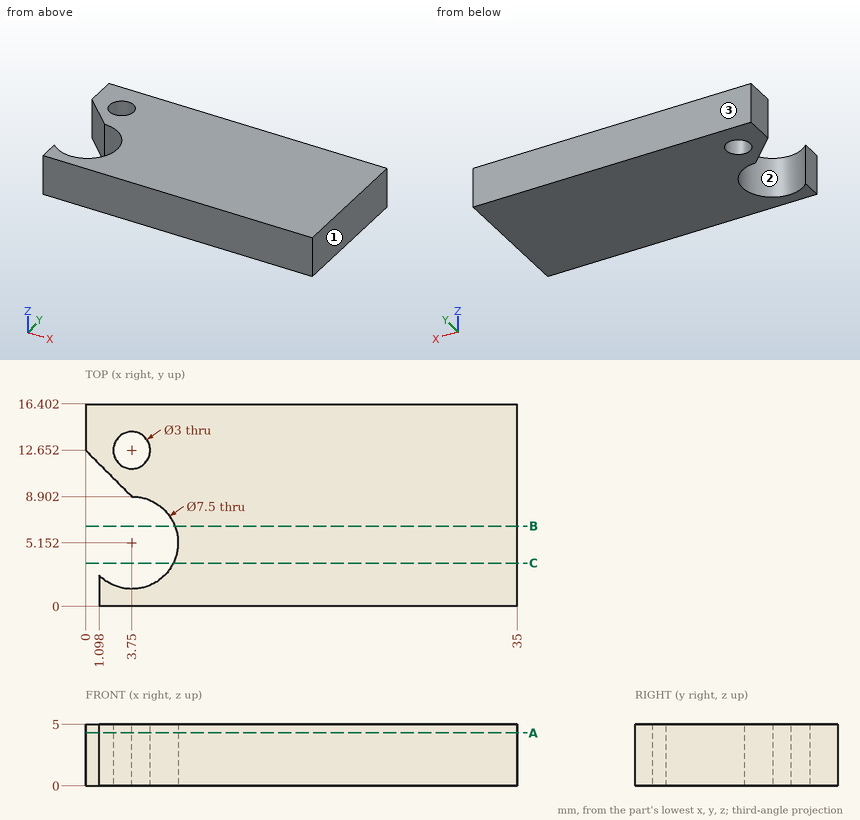
Geometry: see drawing. Coordinates: mm, zero at the bounding-box minimum. Coordinates: 2 decimals unless noted, no trailing zeros. Order: outer loops, then holes, each group sorted by start corner. A loop starts at its lowest first (then second) coordinate and runs counter-clockwise, first axis right, second up. Notation, with made-up numbers: (47.5, 27) - (84.5, 27) arc R27 cw to (84.5, 49) - close; hole circle Ø6 at (48.25, 63). An arc over 180 degrees is marked (long way). Write each question's results on one line, items separated by ' | '.
1) Section B-B, the plane y = 6.5. Return loops of the section in (x, z).
Results list:
outline: (7.25, 0) - (35, 0) - (35, 5) - (7.25, 5) - close
2) Pin query (flat end, axial travel): pin 1 (6 mm diameter, centred on x = 3.75, y = 5.15, fed in from +Z); pin 2 (2 mm diameter, centred on y = 1.5, z = 3, fed in from -X). Return the tip coordinate at first contact, or that it passes through.
Results list:
pin 1: through | pin 2: x = 1.1
3) Line query: line 1 (Y direction, x = 3.75, z = 3.65); line 2 (X direction, y = 12.75, z = 2.8); line 3 (Y direction, x = 4, z = 0.7). Output: solid intervals per line, ascending. Write a range as from..to.
Results list:
line 1: 0..1.4, 8.9..11.15, 14.15..16.4 | line 2: 0..2.25, 5.25..35 | line 3: 0..1.41, 8.89..11.17, 14.13..16.4
4) Section C-C, the plane y = 3.5. Return loops of the section in (x, z).
Results list:
outline: (7.12, 0) - (35, 0) - (35, 5) - (7.12, 5) - close
5) Section A-A, the plane z = 4.3. Return loops of the section in (x, y).
Results list:
outline: (0, 12.65) - (3.75, 8.9) arc R3.75 cw (long way) to (1.1, 2.5) - (1.1, 0) - (35, 0) - (35, 16.4) - (0, 16.4) - close; hole circle Ø3 at (3.75, 12.65)
6) Pull-direction query (X, two-part tool) for the marked faces 1, 2 and 3; classes: pulls with the +X half, pulls with the -X half, needs draft (parallel to the pull), parting line crosses it, or undercut.
Results list:
face 1: pulls with the +X half | face 2: undercut | face 3: needs draft
